Model file for the job. Use its own axes, mm. Face numbers are marked on the shaded views. Coordinates: 2 decimals unless noted, no trailing zeros. Write each loop counter-clockwise with the first axis right and the second up, starting at its lowest first coordinate (ties: lowest second). Pieces come first, ordered by that corner, then holes. Notation, with made-up numbers: M 73,74.5 L 132,74.5 A20 ccw 132,80.5 Z; hole C -26,-1.75 d5. An arc over 180 degrees is marked long. Put each result on its own line as item: value. Start each with the question number.
Q1. Pull direction X, two halves, no side cores. Call the marked faces 1, 2 and 3: pulls with the +X half, pulls with the -X half, needs draft (parallel to the pull), parting line crosses it, or undercut.
Q2. Cut at A-A (z = -1.75). Write the cut outline in (x, y) (3 decimals), then the cut area to 3 significant figures.
Q3. Drill centre lines: line 1 along Y through (x, z) = (-16, -4); line 2 along X through (y, z) = (18, -3.5); line 3 along Y through (x, z) = (0, -2.2) (3 decimals). Where is each one in solid material? Low to high.
Q4. Cut at B-B (y = -14). Write the cut outline in (x, z) (3 decimals), then the cut area to 3 significant figures.
Q5. Cut at C-C (x = 0). Write the cut outline in (y, z) (3 decimals), then the cut area to 3 significant figures.
```python
from build123d import *

# Parameters (mm, degrees)
BASE_SKETCH_W           = 44.45
BASE_SKETCH_H           = 44.45
BASE_SKETCH_R           = 12.7
BASE_EXTRUDE_DEPTH      = 6.35
CORNER_FILLET_R         = 6.35
PERIPHERAL_CHAMFER_SIZE = 0.762
CORNER_SKETCH_R         = 3.3782
CORNER_CUT_DEPTH        = 33.065928179


with BuildPart() as part:
    # Base Sketch → Base Extrude (new body)
    with BuildSketch(Plane.XY):
        Rectangle(BASE_SKETCH_W, BASE_SKETCH_H)
        Circle(BASE_SKETCH_R, mode=Mode.SUBTRACT)
    extrude(amount=-BASE_EXTRUDE_DEPTH)

    # Corner Fillet
    corner_fillet_edges = [part.edges().sort_by_distance(p)[0] for p in [
        (-22.225, 22.225, -3.175),
        (22.225, 22.225, -3.175),
        (22.225, -22.225, -3.175),
        (-22.225, -22.225, -3.175),
    ]]
    fillet(corner_fillet_edges, radius=CORNER_FILLET_R)

    # Peripheral Chamfer
    peripheral_chamfer_edges = [part.edges().sort_by_distance(p)[0] for p in [
        (-12.7, 0, -6.35),
        (-12.7, 0, 0),
        (-22.225, 0, 0),
        (-22.225, 0, -6.35),
        (0, -22.225, 0),
        (22.225, 0, 0),
        (0, 22.225, 0),
        (20.365128061, 20.365128061, 0),
        (20.365128061, -20.365128061, 0),
        (-20.365128061, 20.365128061, 0),
        (-20.365128061, -20.365128061, 0),
        (0, -22.225, -6.35),
        (0, 22.225, -6.35),
        (22.225, 0, -6.35),
        (20.365128061, 20.365128061, -6.35),
        (20.365128061, -20.365128061, -6.35),
        (-20.365128061, 20.365128061, -6.35),
        (-20.365128061, -20.365128061, -6.35),
    ]]
    chamfer(peripheral_chamfer_edges, length=PERIPHERAL_CHAMFER_SIZE)

    # Corner Sketch → Corner Cut (cut, through all)
    with BuildSketch(Plane.XY):
        with Locations((15.875, 15.875)):
            Circle(CORNER_SKETCH_R)
        with Locations((15.875, -15.875)):
            Circle(CORNER_SKETCH_R)
        with Locations((-15.875, -15.875)):
            Circle(CORNER_SKETCH_R)
        with Locations((-15.875, 15.875)):
            Circle(CORNER_SKETCH_R)
    extrude(amount=-CORNER_CUT_DEPTH, mode=Mode.SUBTRACT)


solid = part.part
```
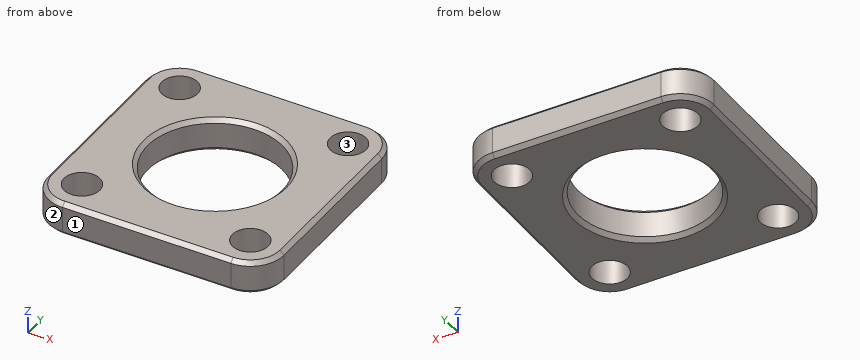
Computed values:
1. face 1: needs draft
1. face 2: pulls with the -X half
1. face 3: undercut
2. outline: M -22.225,-15.875 A6.35 ccw -15.875,-22.225 L 15.875,-22.225 A6.35 ccw 22.225,-15.875 L 22.225,15.875 A6.35 ccw 15.875,22.225 L -15.875,22.225 A6.35 ccw -22.225,15.875 Z; hole C -15.875,-15.875 d6.756; hole C -15.875,15.875 d6.756; hole C 0,0 d25.4; hole C 15.875,-15.875 d6.756; hole C 15.875,15.875 d6.756
2. area: 1,290 mm2
3. line 1: -22.22 to -19.25, -12.5 to 12.5, 19.25 to 22.22
3. line 2: -21.86 to -18.5, -13.25 to 13.25, 18.5 to 21.86
3. line 3: -22.225 to -12.7, 12.7 to 22.225
4. outline: M -22.225,-5.588 L -21.463,-6.35 L -18.685,-6.35 L -18.685,0 L -21.463,0 L -22.225,-0.762 Z; M -13.065,-6.35 L 13.065,-6.35 L 13.065,0 L -13.065,0 Z; M 18.685,-6.35 L 21.463,-6.35 L 22.225,-5.588 L 22.225,-0.762 L 21.463,0 L 18.685,0 Z
4. area: 210 mm2
5. outline: M -22.225,-5.588 L -21.463,-6.35 L -13.462,-6.35 L -12.7,-5.588 L -12.7,-0.762 L -13.462,0 L -21.463,0 L -22.225,-0.762 Z; M 12.7,-5.588 L 13.462,-6.35 L 21.463,-6.35 L 22.225,-5.588 L 22.225,-0.762 L 21.463,0 L 13.462,0 L 12.7,-0.762 Z
5. area: 119 mm2
